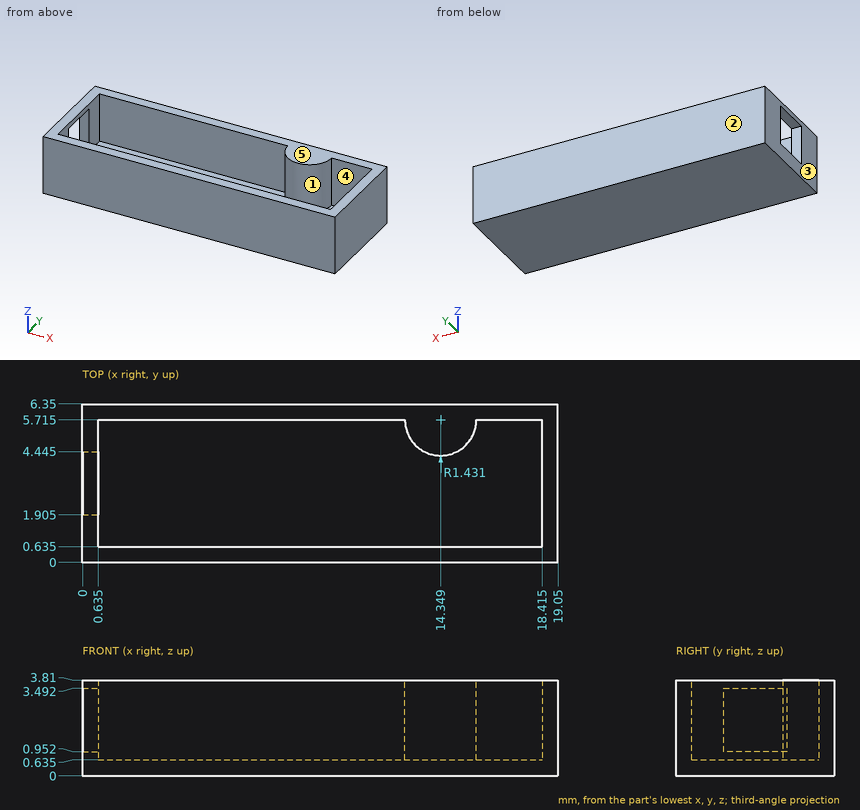
Check sheet for the drawn part. Datum: minimum x, y, z corner. Units: mm. A direction names the side the tool comes from. Round coordinates to 2 decimals unless told otherwise and drop trailing zeros. Write item = value, one per line. Start each with the question number.
1. Mould release check, pull along Y, two halves, no side actions. Record for the marked faces 1, 2 and 3: released by +Y, released by -Y, zero draft, split by the parting line, or undercut.
2. Thickness scan on line 1 (Z direction, x = 4.75, y = 2.5) (1 decimal). Record the ranges inside material, lowest first.
3. Set-up check for the marked faces 4 and 5: record each of +Z, -Z, +X, -X, +Y, -Y from which the full face is reachable in a straight line by a thin tool's end or side.
4. Depth check by flat-ended pin: pin 1 (2.5 mm diameter, centred on x = 11.5, y = 3, fed in from +Z) (1 decimal). Enter the tip coordinate at first touch or a pass-through.
Working result:
q1.face_1 = undercut
q1.face_2 = released by +Y
q1.face_3 = zero draft
q2.line_1 = 0 to 0.6
q3.face_4 = +Z
q3.face_5 = +Z, +X, -X, +Y, -Y
q4.pin_1 = 0.6
